Verification items for this drawing (mm, ordinates from the low corner). Coordinates: 2 decimals unless noted, no trailing zeros. Order: outer loops, then holes, each group sorted by start corner. A loop starts at its lowest first (then second) coordinate and runs counter-clockwise, first axis right, second up. Notation, with made-up numbers: (40, 6.25) -> (97, 6.25) arc R13 cw to (97, 21.25) -> close; hole circle Ø10 at (88.25, -4.5). An arc over 180 degrees is marked (long way). Write item = value, one per line. Start each with the question number.
1. Thickness scan on line 1 along X through (y, z) = (48, 7.25); line 2 along Y through (x, z) = (60.5, 8); line 3 along Y through (x, z) = (27.5, 6). Record the ranges inside material, lowest first. Write a range as from..to.
2. Cross-section at D-D on x = 5. Record the cut outline in (y, z).
3. Cross-section at A-A on x = 13. Record the cut outline in (y, z).
4. Cross-section at C-C on y = 39.5. Record the cut outline in (x, z).
5. Cross-section at B-B on z = 7. Record the cut outline in (x, y), plus the area to 3 significant figures.
6. Go/stop test with flat-tipped pins: P1, Ø9, axis at x = 45, y = 5.5, coming from the +Z side; P2, Ø4, axis at y = 55, z = 4, coming from the -X side; P3, Ø5.5, axis at x = 36, y = 6, coming from the -Z side; P4, Ø3, axis at x = 13, y = 33.5, coming from the -Z side. Record where each tip stops, or that it passes through.
7. Release check for a two-part mould opening along X. For the marked faces 1 and 2 record: +X half, -X half, draft (parallel to the pull), parting line (faces both ways), or undercut.
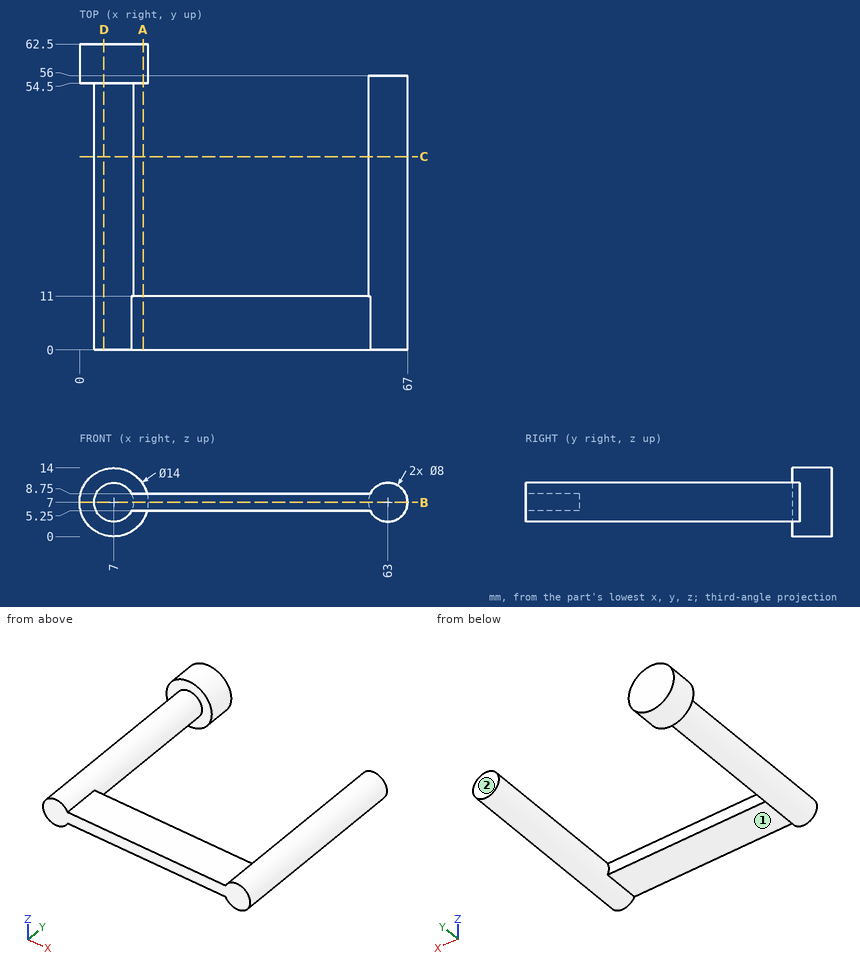
Worked out:
q1.line_1 = 3.01..10.99, 59.01..66.99
q1.line_2 = 0..56
q1.line_3 = 0..11
q2.outline = (0, 3.54) -> (54.5, 3.54) -> (54.5, 0.29) -> (62.5, 0.29) -> (62.5, 13.71) -> (54.5, 13.71) -> (54.5, 10.46) -> (0, 10.46) -> close
q3.outline = (0, 5.25) -> (11, 5.25) -> (11, 8.75) -> (0, 8.75) -> close; (54.5, 3.39) -> (62.5, 3.39) -> (62.5, 10.61) -> (54.5, 10.61) -> close
q4.outline = circle Ø8 at (7, 7); circle Ø8 at (63, 7)
q5.outline = (0, 54.5) -> (3, 54.5) -> (3, 0) -> (67, 0) -> (67, 56) -> (59, 56) -> (59, 11) -> (11, 11) -> (11, 54.5) -> (14, 54.5) -> (14, 62.5) -> (0, 62.5) -> close
q5.area = 1,520 mm²
q6.P1 = 8.75
q6.P2 = 0.07
q6.P3 = 5.25
q6.P4 = through
q7.face_1 = undercut
q7.face_2 = draft
